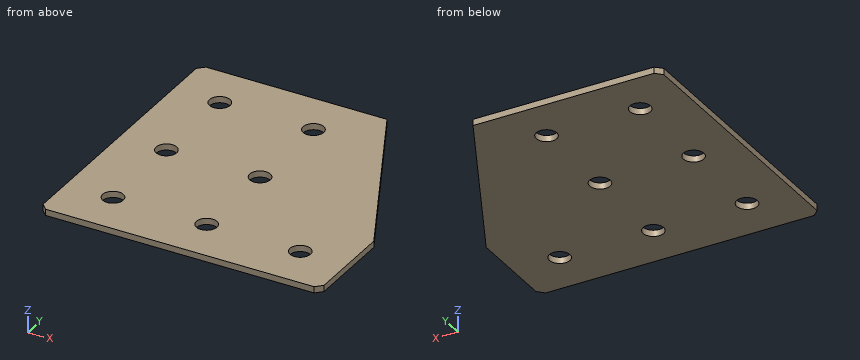
```python
from build123d import *

# Parameters (mm, degrees)
EXTRUDE_1_DEPTH   = 2
HOLE_WIZARD_M61_D = 6.6
CHAMFER_1_SIZE    = 2


with BuildPart() as part:
    # Эскиз1 → Бобышка-Вытянуть1 (new body)
    with BuildSketch(Plane(origin=(0, 0, 0), x_dir=(1, 0, 0), z_dir=(0, 0, -1))):
        Polygon((0, 0), (0, 90), (90, 90), (90, 60), (60, 0), align=None)
    extrude(amount=EXTRUDE_1_DEPTH)

    # Отверстие с зазором M61 (through all)
    with Locations(Plane(origin=(0, 0, -2), x_dir=(1, 0, 0), z_dir=(0, 0, -1))):
        with Locations((45, 75), (15, 75), (15, 45), (15, 15), (75, 75), (45, 45), (45, 15)):
            Hole(HOLE_WIZARD_M61_D / 2)

    # Фаска1
    chamfer_1_edges = [part.edges().sort_by_distance(p)[0] for p in [
        (0, 0, -1),
        (0, -90, -1),
        (90, -90, -1),
    ]]
    chamfer(chamfer_1_edges, length=CHAMFER_1_SIZE)


solid = part.part
```
Build history of the part. All positions in model axes, mm. Give positions to 0.01 mm unless a question says otherwise; leave off trailing zeros. Loops run counter-clockwise (first coordinate to the right, second up) from the corner with the lowest first, then second, coordinate; pieces in that order, holes last.
Item 1: Drill centre lines: line 1 (Y direction, x = 45, z = -1.5); line 2 (X direction, y = -75, z = -0.6); line 3 (Y direction, x = 16, z = -1.65). Where is each one in solid material? Low to high.
Answers follow:
line 1: y = -90 to -78.3, -71.7 to -48.3, -41.7 to -18.3, -11.7 to 0
line 2: x = 0 to 11.7, 18.3 to 41.7, 48.3 to 71.7, 78.3 to 90
line 3: y = -90 to -78.14, -71.86 to -48.14, -41.86 to -18.14, -11.86 to 0
Item 2: Slice it at B-B, the plane x = 75. List the corners of the cut face in (y, z), and give its area (3 significant figures).
Answers follow:
outline: (-90, -2) - (-78.3, -2) - (-78.3, 0) - (-90, 0) - close; (-71.7, -2) - (-30, -2) - (-30, 0) - (-71.7, 0) - close
area: 107 mm2
Item 3: Slice it at C-C, the plane y = -45. List the corners of the cut face in (x, z).
Answers follow:
outline: (0, -2) - (11.7, -2) - (11.7, 0) - (0, 0) - close; (18.3, -2) - (41.7, -2) - (41.7, 0) - (18.3, 0) - close; (48.3, -2) - (82.5, -2) - (82.5, 0) - (48.3, 0) - close
Item 4: Slice it at A-A, the plane y = -75. List the corners of the cut face in (x, z).
Answers follow:
outline: (0, -2) - (11.7, -2) - (11.7, 0) - (0, 0) - close; (18.3, -2) - (41.7, -2) - (41.7, 0) - (18.3, 0) - close; (48.3, -2) - (71.7, -2) - (71.7, 0) - (48.3, 0) - close; (78.3, -2) - (90, -2) - (90, 0) - (78.3, 0) - close
Item 5: Flat gauge pin, fed straight in: pin 1 (6 mm diameter, centred on x = 15, y = -75, fed in from -Z). Where does the tip first touch, or does it go through?
Answers follow:
pin 1: passes through
Item 6: Slice it at D-D, the plane z = -1. List the corners of the cut face in (x, y), and give its area (3 significant figures).
Answers follow:
outline: (0, -88) - (2, -90) - (88, -90) - (90, -88) - (90, -60) - (60, 0) - (2, 0) - (0, -2) - close; hole circle Ø6.6 at (15, -75); hole circle Ø6.6 at (15, -45); hole circle Ø6.6 at (15, -15); hole circle Ø6.6 at (45, -75); hole circle Ø6.6 at (45, -45); hole circle Ø6.6 at (45, -15); hole circle Ø6.6 at (75, -75)
area: 6,950 mm2
